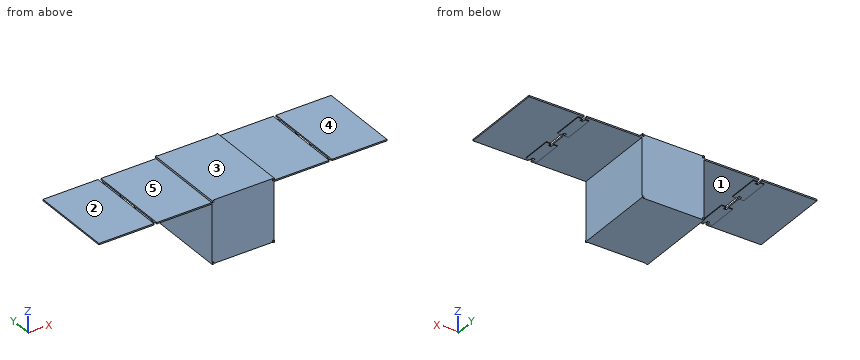
```python
from build123d import *

# Parameters (mm, degrees)
ESTRUSIONE_ESTRUSIONE2_DEPTH      = 150
ESTRUSIONE_ESTRUSIONE2_DEPTH_BACK = 150
ESTRUSIONE_ESTRUSIONE3_DEPTH      = 3.3
ESTRUSIONE_ESTRUSIONE3_DEPTH_BACK = 303.3
SCHIZZO3_W                        = 6.5
SCHIZZO3_H                        = 6.5
SCHIZZO5_W                        = 5
SCHIZZO5_H                        = 300
ESTRUSIONE_ESTRUSIONE4_DEPTH      = 200
SCHIZZO6_W                        = 15
SCHIZZO6_H                        = 110
SCHIZZO6_W_2                      = 25
ESTRUSIONE_ESTRUSIONE5_DEPTH      = 2.5
SCHIZZO7_W                        = 10
SCHIZZO7_H                        = 12
TAGLIO_ESTRUSIONE1_DEPTH          = 2.5
SCHIZZO8_W                        = 200
SCHIZZO8_H                        = 300
ESTRUSIONE_ESTRUSIONE6_DEPTH      = 5
SCHIZZO11_W                       = 5
SCHIZZO11_H                       = 300
ESTRUSIONE_ESTRUSIONE8_DEPTH      = 200
SCHIZZO12_W                       = 40
SCHIZZO12_H                       = 110
ESTRUSIONE_ESTRUSIONE9_DEPTH      = 2.5
SCHIZZO13_W                       = 10
SCHIZZO13_H                       = 12
TAGLIO_ESTRUSIONE2_DEPTH          = 2.5
SCHIZZO14_W                       = 200
SCHIZZO14_H                       = 300
ESTRUSIONE_ESTRUSIONE10_DEPTH     = 5


with BuildPart() as part:
    # Schizzo2 → Estrusione-Estrusione2 (new, two sides: drawn at the far end of the back side and taken through both)
    with BuildSketch(Plane(origin=(0, 0, 0), x_dir=(1, 0, 0), z_dir=(0, 1, 0)).offset(-ESTRUSIONE_ESTRUSIONE2_DEPTH_BACK)):
        Polygon((-113.15, 106.65), (-113.15, -106.65), (-106.65, -106.65), (-106.65, -113.15), (106.65, -113.15), (106.65, -106.65), (113.15, -106.65), (113.15, 106.65), (106.65, 106.65), (106.65, 113.15), (-106.65, 113.15), (-106.65, 106.65), align=None)
    extrude(amount=ESTRUSIONE_ESTRUSIONE2_DEPTH + ESTRUSIONE_ESTRUSIONE2_DEPTH_BACK)

    # Schizzo3 → Estrusione-Estrusione3 (add, two sides: drawn at the far end of the back side and taken through both)
    with BuildSketch(Plane.XZ.offset(150).offset(-ESTRUSIONE_ESTRUSIONE3_DEPTH_BACK)):
        with Locations((-109.9, 109.9)):
            Rectangle(SCHIZZO3_W, SCHIZZO3_H)
        with Locations((109.9, 109.9)):
            Rectangle(SCHIZZO3_W, SCHIZZO3_H)
        with Locations((109.9, -109.9)):
            Rectangle(SCHIZZO3_W, SCHIZZO3_H)
        with Locations((-109.9, -109.9)):
            Rectangle(SCHIZZO3_W, SCHIZZO3_H)
    extrude(amount=ESTRUSIONE_ESTRUSIONE3_DEPTH + ESTRUSIONE_ESTRUSIONE3_DEPTH_BACK)

    # Schizzo5 → Estrusione-Estrusione4 (add)
    with BuildSketch(Plane.ZY.offset(113.15)):
        with Locations((103.15, 0)):
            Rectangle(SCHIZZO5_W, SCHIZZO5_H)
    extrude(amount=ESTRUSIONE_ESTRUSIONE4_DEPTH)

    # Schizzo6 → Estrusione-Estrusione5 (add)
    with BuildSketch(Plane(origin=(0, 0, 100.65), x_dir=(-1, 0, 0), z_dir=(0, 0, -1))):
        with Locations((305.65, 85)):
            Rectangle(SCHIZZO6_W, SCHIZZO6_H)
        with Locations((325.65, 85)):
            Rectangle(SCHIZZO6_W_2, SCHIZZO6_H)
        with Locations((305.65, -85)):
            Rectangle(SCHIZZO6_W, SCHIZZO6_H)
        with Locations((325.65, -85)):
            Rectangle(SCHIZZO6_W_2, SCHIZZO6_H)
    extrude(amount=ESTRUSIONE_ESTRUSIONE5_DEPTH)

    # Schizzo7 → Taglio-Estrusione1 (cut)
    with BuildSketch(Plane.XY.offset(100.65)):
        with Locations((-318.15, 134)):
            Rectangle(SCHIZZO7_W, SCHIZZO7_H)
        with Locations((-318.15, 36)):
            Rectangle(SCHIZZO7_W, SCHIZZO7_H)
        with Locations((-318.15, -36)):
            Rectangle(SCHIZZO7_W, SCHIZZO7_H)
        with Locations((-318.15, -134)):
            Rectangle(SCHIZZO7_W, SCHIZZO7_H)
    extrude(amount=-TAGLIO_ESTRUSIONE1_DEPTH, mode=Mode.SUBTRACT)

    # Schizzo8 → Estrusione-Estrusione6 (add)
    with BuildSketch(Plane.XY.offset(100.65)):
        with Locations((-423.15, 0)):
            Rectangle(SCHIZZO8_W, SCHIZZO8_H)
    extrude(amount=ESTRUSIONE_ESTRUSIONE6_DEPTH)

    # Schizzo11 → Estrusione-Estrusione8 (add)
    with BuildSketch(Plane(origin=(113.15, 0, 0), x_dir=(0, 0, -1), z_dir=(1, 0, 0))):
        with Locations((-103.15, 0)):
            Rectangle(SCHIZZO11_W, SCHIZZO11_H)
    extrude(amount=ESTRUSIONE_ESTRUSIONE8_DEPTH)

    # Schizzo12 → Estrusione-Estrusione9 (add)
    with BuildSketch(Plane(origin=(0, 0, 100.65), x_dir=(-1, 0, 0), z_dir=(0, 0, -1))):
        with Locations((-318.15, 85)):
            Rectangle(SCHIZZO12_W, SCHIZZO12_H)
        with Locations((-318.15, -85)):
            Rectangle(SCHIZZO12_W, SCHIZZO12_H)
    extrude(amount=ESTRUSIONE_ESTRUSIONE9_DEPTH)

    # Schizzo13 → Taglio-Estrusione2 (cut)
    with BuildSketch(Plane(origin=(0, 0, 98.15), x_dir=(-1, 0, 0), z_dir=(0, 0, -1))):
        with Locations((-318.15, 134)):
            Rectangle(SCHIZZO13_W, SCHIZZO13_H)
        with Locations((-318.15, 36)):
            Rectangle(SCHIZZO13_W, SCHIZZO13_H)
        with Locations((-318.15, -36)):
            Rectangle(SCHIZZO13_W, SCHIZZO13_H)
        with Locations((-318.15, -134)):
            Rectangle(SCHIZZO13_W, SCHIZZO13_H)
    extrude(amount=-TAGLIO_ESTRUSIONE2_DEPTH, mode=Mode.SUBTRACT)

    # Schizzo14 → Estrusione-Estrusione10 (add)
    with BuildSketch(Plane.XY.offset(100.65)):
        with Locations((423.15, 0)):
            Rectangle(SCHIZZO14_W, SCHIZZO14_H)
    extrude(amount=ESTRUSIONE_ESTRUSIONE10_DEPTH)


solid = part.part
```
Check sheet for the modelled part. Datum: model origin and axes. Units: mm. Face numbers are marked on the shaded views. A direction names the side the tool comes from. Coordinates: 2 decimals unless noted, no trailing zeros. Loops run counter-clockwise (first coordinate to the right, second up) from the corner with the lowest first, then second, coordinate; pieces in that order, holes last.
1) Material ranges on probe 1 along Y at (x, z) = (89, 32.5); probe 2 along Z at (x, y) = (-301, 102); probe 3 along X at (y, z) = (-65.5, 73), recorded low to high.
2) Sectioned sample at D-D (y = -96.5). Record the boundary of the cut face in (x, z), and give its area (3 significant figures).
3) Sectioned sample at C-C (z = -42). Record the boundary of the cut face in (x, y).
4) Access from +Z, -Z, +X, -X, +Y, -Y to the whole of each face (thin tool, end or side, straight path). Record for the marked faces 3, 4 and 5.
5) Gauge pin test, flat ends, axial feed: pin 1 (1.2 mm diameter, centred on x = 320.5, z = 99, fed in from -Y); pin 2 (1 mm diameter, centred on y = -151.5, z = -110, fed in from +X); pin 3 (12 mm diameter, centred on x = 376.5, y = -47, fed in from +Z). Record the tip position at first contact, or that the pin passes through.
6) Sectioned sample at A-A (y = 8). Record the boundary of the cut face in (x, z), and give its area (3 significant figures).
7) Sectioned sample at B-B (x = 92). Record the boundary of the cut face in (y, z).
8) Release check for a two-part mould opening along X. For the marked faces 1 and 2 record: released by +X, released by -X, zero draft, split by the parting line, or undercut.
Check sheet entries:
1. probe 1: y = -150 to 150
1. probe 2: z = 98.15 to 105.65
1. probe 3: x = -113.15 to 113.15
2. outline: (-523.15, 100.65) - (-338.15, 100.65) - (-338.15, 98.15) - (-298.15, 98.15) - (-298.15, 100.65) - (-113.15, 100.65) - (-113.15, -113.15) - (113.15, -113.15) - (113.15, 100.65) - (298.15, 100.65) - (298.15, 98.15) - (338.15, 98.15) - (338.15, 100.65) - (523.15, 100.65) - (523.15, 105.65) - (323.15, 105.65) - (323.15, 100.65) - (313.15, 100.65) - (313.15, 105.65) - (113.15, 105.65) - (113.15, 113.15) - (-113.15, 113.15) - (-113.15, 105.65) - (-313.15, 105.65) - (-313.15, 100.65) - (-323.15, 100.65) - (-323.15, 105.65) - (-523.15, 105.65) - close
2. area: 55,400 mm2
3. outline: (-113.15, -150) - (113.15, -150) - (113.15, 150) - (-113.15, 150) - close
4. face 3: +Z, +X, -X, +Y, -Y
4. face 4: +Z, +X, +Y, -Y
4. face 5: +Z, -X, +Y, -Y
5. pin 1: stops at y = -128
5. pin 2: stops at x = 113.15
5. pin 3: stops at z = 105.65
6. outline: (-523.15, 100.65) - (-323.15, 100.65) - (-323.15, 105.65) - (-523.15, 105.65) - close; (-313.15, 100.65) - (-113.15, 100.65) - (-113.15, -113.15) - (113.15, -113.15) - (113.15, 100.65) - (313.15, 100.65) - (313.15, 105.65) - (113.15, 105.65) - (113.15, 113.15) - (-113.15, 113.15) - (-113.15, 105.65) - (-313.15, 105.65) - close; (323.15, 100.65) - (523.15, 100.65) - (523.15, 105.65) - (323.15, 105.65) - close
6. area: 55,200 mm2
7. outline: (-150, -113.15) - (150, -113.15) - (150, 113.15) - (-150, 113.15) - close
8. face 1: undercut
8. face 2: zero draft
